Part model, mm, in its own coordinate system. Round coordinates to 2 decimals unless told otherwise and drop trailing zeros. Loops run counter-clockwise (first coordinate to the right, second up) from the corner with the lowest first, then second, coordinate; pieces in that order, holes last. Notation, with made-up numbers: (32, 16.5) -> (36, 16.5) arc R27 ccw to (36, 46.5) -> close; hole circle Ø8 at (22.25, 41). An arc over 180 degrees is marked (long way). Use a Markdown table: item, result. Add a question column.
Item 1: Cut at C-C, the plane z = 184.5. State how many separate pieces and enclosed holes the cut face has, plus the area to 3 significant figures.
Item 2: Cut at B-B, the plane x = -147. List the corners of the cut face in (y, z), plus the area to 3 significant figures.
Item 3: Probe line 1 (X direction, y = -24, z = 185.65); line 2 (Y direction, x = 34.5, z = 185.6); line 3 (Y direction, x = -74.5, z = 186.9). List the from-to ranges inside material, lowest first. Write a range as [from, to].
Item 4: Cut at A-A, the plane y = -46. List the corners of the cut face in (x, z), plus the area to 3 significant figures.
Item 5: Flat gauge pins, fed straight in: pin 1 (0.9 mm diameter, centred on x = -41, z = 185.5, fed in from -Y); pin 2 (1.1 mm diameter, centred on y = 33.5, z = 185.5, fed in from -X). Where does each tip first touch, or does it go through?
```python
from build123d import *

# Parameters (mm, degrees)
SKETCH2_W           = 230
SKETCH2_H           = 216
BOSS_EXTRUDE1_DEPTH = 3
SKETCH5_W           = 190
SKETCH5_H           = 137.85
SKETCH5_W_2         = 10.3
SKETCH5_H_2         = 2.3
SKETCH5_W_3         = 2.3
SKETCH5_H_3         = 56.3
CUT_EXTRUDE3_DEPTH  = 3


with BuildPart() as part:
    # Sketch2 → Boss-Extrude1 (new body)
    with BuildSketch(Plane.XY.offset(184)):
        with Locations((-57.5, 0)):
            Rectangle(SKETCH2_W, SKETCH2_H)
    extrude(amount=BOSS_EXTRUDE1_DEPTH)

    # Sketch5 → Cut-Extrude3 (cut)
    with BuildSketch(Plane.XY.offset(187)):
        with Locations((-56.65, -39.075)):
            Rectangle(SKETCH5_W, SKETCH5_H)
        with Locations((32.5, 34)):
            Rectangle(SKETCH5_W_2, SKETCH5_H_2)
        with Locations((52.5, 34)):
            Rectangle(SKETCH5_W_2, SKETCH5_H_2)
        with Locations((42.5, 0)):
            Rectangle(SKETCH5_W_3, SKETCH5_H_3)
        with Locations((52.5, -34)):
            Rectangle(SKETCH5_W_2, SKETCH5_H_2)
        with Locations((-157.5, 0)):
            Rectangle(SKETCH5_W_3, SKETCH5_H_3)
        with Locations((-147.5, 34)):
            Rectangle(SKETCH5_W_2, SKETCH5_H_2)
        with Locations((-167.5, 34)):
            Rectangle(SKETCH5_W_2, SKETCH5_H_2)
        with Locations((-167.5, -34)):
            Rectangle(SKETCH5_W_2, SKETCH5_H_2)
    extrude(amount=-CUT_EXTRUDE3_DEPTH, mode=Mode.SUBTRACT)


solid = part.part
```
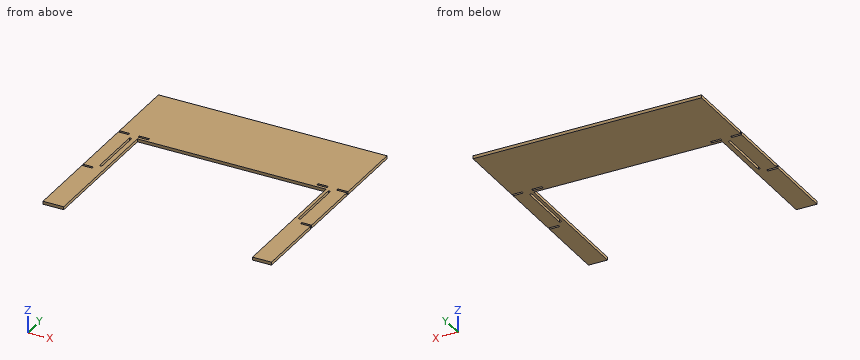
A:
| question | item | result |
|---|---|---|
| 1 | separate pieces | 1 |
| 1 | enclosed holes | 4 |
| 1 | area | 23,100 mm^2 |
| 2 | outline | (29.85, 184) -> (32.85, 184) -> (32.85, 187) -> (29.85, 187) -> close; (35.15, 184) -> (108, 184) -> (108, 187) -> (35.15, 187) -> close |
| 2 | area | 228 mm^2 |
| 3 | line 1 | x = [-172.5, -158.65], [-156.35, -151.65], [38.35, 41.35], [43.65, 57.5] |
| 3 | line 2 | y = [29.85, 32.85], [35.15, 108] |
| 3 | line 3 | y = [29.85, 108] |
| 4 | outline | (-172.5, 184) -> (-151.65, 184) -> (-151.65, 187) -> (-172.5, 187) -> close; (38.35, 184) -> (57.5, 184) -> (57.5, 187) -> (38.35, 187) -> close |
| 4 | area | 120 mm^2 |
| 5 | pin 1 | stops at y = 29.85 |
| 5 | pin 2 | stops at x = -162.35 |
